Autodesk Inventor part; units mm, degrees
ref_plane "YZ Plane" through (0, 0, 0) normal (1, 0, 0) x (0, 1, 0)
ref_plane "XZ Plane" through (0, 0, 0) normal (0, 1, 0) x (-1, 0, 0)
ref_plane "XY Plane" through (0, 0, 0) normal (0, 0, 1) x (1, 0, 0)
sketch "Sketch1" plane through (0, 0, 0) normal (0, 0, 1) x (1, 0, 0)
  line L0 (-19, -13) -> (19, -13)
  line L1 (19, -13) -> (19, 13)
  line L2 (19, 13) -> (-19, 13)
  line L3 (-19, 13) -> (-19, -13)
  line L4 (-19, -13) -> (19, 13) construction
  line L5 (19, -13) -> (-19, 13) construction
  point P0 (0, 0)
  dimension "d0" = 26
  dimension "d1" = 38
extrude "Extrusion1" add sketch "Sketch1" along normal blind 20
sketch "Sketch2" plane through (0, 0, 20) normal (0, 0, 1) x (1, 0, 0)
  line L0 (-26.6, 0) -> (26.6, 0)
  line L1 (-19, 10) -> (10, 10)
  line L2 (10, 10) -> (10, -10)
  line L3 (10, -10) -> (-19, -10)
  line L4 (-19, -10) -> (-19, 10)
  line L5 (-19, 10) -> (10, -10) construction
  line L6 (10, 10) -> (-19, -10) construction
  line L7 (19, 13) -> (-19, 13)
  line L8 (19, -13) -> (19, 13)
  line L9 (-19, 13) -> (-19, -13)
  line L10 (10, 10) -> (16, 10)
  line L11 (16, 10) -> (16, -10)
  line L12 (16, -10) -> (10, -10)
  line L13 (10, -10) -> (10, 10)
  point P0 (0, 0)
  point P1 (-4.5, 0)
  point P2 (-19, 0)
  dimension "d5" = 20
  dimension "d7" = 29
  dimension "d8" = 9
  dimension "d9" = 3
extrude "Extrusion2" cut sketch "Sketch2" against normal blind 15 contours L4 L1 L2 L0 | L0 L2 L3 L4 | L2 L10 L11 L0 | L0 L11 L12 L2
sketch "Sketch3" plane through (0, 0, 5) normal (0, 0, 1) x (1, 0, 0)
  line L0 (-26.6, 0) -> (26.6, 0)
  circle A0 centre (-4.5, 0) radius 9
  line L1 (-19, -10) -> (-19, 10)
  point P0 (0, 0)
  dimension "d12" = 18
  dimension "d13" = 14.5
extrude "Extrusion3" cut sketch "Sketch3" against normal blind 2.5
sketch "Sketch4" plane through (-4.5, 0, 2.5) normal (0, 0, 1) x (1, 0, 0)
  circle A0 centre (0, 0) radius 9
  circle A1 centre (0, 0) radius 6.25
  point P0 (4.5, 0)
  dimension "d16" = 12.5
extrude "Extrusion4" cut sketch "Sketch4" against normal blind 2.5 contours A1
chamfer "Chamfer1" distance 1 angle 45 1 edges at (-13.5, 0, 5)
chamfer "Chamfer2" distance 1 angle 45 1 edges at (-10.75, 0, 2.5)
chamfer "Chamfer3" distance 2.5 angle 45 2 edges at (16, -10, 12.5) (16, 10, 12.5)
chamfer "Chamfer5" distance 1 angle 45 1 edges at (16, 0, 5)
sketch "Sketch5" plane through (16, -7.5, 20) normal (-1, 0, 0) x (0, 0, 1)
  line L0 (-24, 7.5) -> (4, 7.5)
  circle A0 centre (-7, 7.5) radius 3
  line L1 (0, 15) -> (0, 0)
  point P0 (-20, 7.5)
  dimension "d34" = 6
  dimension "d35" = 7
extrude "Extrusion5" cut sketch "Sketch5" against normal through all
chamfer "Chamfer6" distance 2.75 angle 45 5 edges at (0, -13, 0) (-19, 0, 0) (0, 13, 0) (-19, 13, 10) (-19, -13, 10)
properties part number "_3DPrint"
Design review of the part built by this model. Coordinates are the model's own, in mm. A direction names the side the tool comes from. Round coordinates to 2 decimals unless told otherwise and drop trailing zeros. Write each loop counter-clockwise with the first axis right and the second up, starting at its lowest first coordinate (ties: lowest second). Pieces come first, ordered by that corner, then holes.
Item 1: For faces 4 (the flat face through (5, 5, 5)), 5 (the flat face through (2, 13, 11)), 6 (the flat face through (-11, 4, 2.5)), list the 3-axis set-ups (+Z, -Z, +X, -X, +Y, -Y) from which the entire face can be reached by the end or side of a thin tool; tool diameter is ignored.
Item 2: We need section D-D on x = 8. Write out the cut boundary in (y, z).
Item 3: We need section A-A on z = 13. Write out the cut boundary in (x, y), and give its area (3 significant figures).
Item 4: For probe 1 along X at (y, z) = (0, 2.85); probe 2 along Y at (x, z) = (1, 15.5); probe 3 along Z at (x, y) = (17.1, 0), list the stretches that pass through material, from the lowest coordinate up.
Item 5: The part is to be moulded in two halves that separate along X. For faces 1 (the flat face through (5, 0, 0)), 2 (the flat face through (-19, 0, 4)), 3 (the cylindrical face through (4.084, 2.703, 3.261)), say which applies: +X half, -X half, draft (parallel to the pull), parting line (faces both ways), or undercut.
Item 6: Clearance check with flat-ended pins moving along their axes: pin 1 Ø5 at (y, z) = (5.5, 17.5) entering from -X; pin 2 Ø4 at (y, z) = (0.5, 10) entering from -X; pin 3 Ø8 at (x, y) = (6, 8) entering from -Z; pin 4 Ø2 at (x, y) = (-13.5, -6) entering from +Z. State where each tip first meets the part, or that it passes through.
Item 7: We need section B-B on y = 0. Write out the cut boundary in (x, z), and give its area (3 significant figures).
Returned:
1. face 4: +Z, -X
1. face 5: +Z, -Z, +X, -X, +Y
1. face 6: +Z
2. outline: (-13, 2.75) - (-10.25, 0) - (10.25, 0) - (13, 2.75) - (13, 20) - (10, 20) - (10, 5) - (-10, 5) - (-10, 20) - (-13, 20) - close
3. outline: (-19, -10.25) - (-16.25, -13) - (19, -13) - (19, -3) - (16, -3) - (16, -7.5) - (13.5, -10) - (-19, -10) - close; (-19, 10) - (13.5, 10) - (16, 7.5) - (16, 3) - (19, 3) - (19, 13) - (-16.25, 13) - (-19, 10.25) - close
3. area: 269 mm2
4. probe 1: x = -19 to -13.5, 4.5 to 19
4. probe 2: y = -13 to -10, 10 to 13
4. probe 3: z = 0 to 10, 16 to 20
5. face 1: draft
5. face 2: -X half
5. face 3: undercut
6. pin 1: stops at x = 15.5
6. pin 2: stops at x = 16
6. pin 3: stops at z = 0
6. pin 4: stops at z = 5
7. outline: (-19, 2.75) - (-16.25, 0) - (-10.75, 0) - (-10.75, 1.5) - (-11.75, 2.5) - (-13.5, 2.5) - (-13.5, 4) - (-14.5, 5) - (-19, 5) - close; (1.75, 0) - (19, 0) - (19, 10) - (16, 10) - (16, 6) - (15, 5) - (5.5, 5) - (4.5, 4) - (4.5, 2.5) - (2.75, 2.5) - (1.75, 1.5) - close; (16, 16) - (19, 16) - (19, 20) - (16, 20) - close
7. area: 135 mm2
